Check sheet for the modelled part. Datum: model origin and axes. Units: mm. A direction names the side the tool comes from. Round coordinates to 2 decimals unless told otherwise and drop trailing zeros. Write each loop counter-clockwise with the first axis right and the second up, starting at its lowest first coordinate (ties: lowest second). Pieces come first, ordered by that corner, then holes.
Item 1: Tool access check on faces 4 (the flat face through (11.5, -23, 128)), 5 (the flat face through (12, -7, 132)), 6 (the cylindrical face through (12.83, 22.73, 128.25)), 7 (the flat face through (22, 0, 167.8)). Record the directions out of +Z, -Z, +X, -X, +Y, -Y that give a thin tool (end or side, any length) a straight path to the whole face; none if there is none.
Item 2: Cross-section at D-D on x = 26. Enter the section's corners in (y, z), plus the area to 3 significant figures.
Item 3: Cross-section at A-A on z = 129.2. Enter the section's corners in (x, y).
Item 4: Release check for a two-part mould opening along Z. For faces 1 (the cylindrical face through (12.83, -21.27, 128.25)), 2 (the flat face through (29.2, 0, 169)), 3 (the flat face through (12, 0, 138.2)) record: +Z half, -Z half, draft (parallel to the pull), parting line (faces both ways), or undercut.
Item 5: Go/stop test with flat-tipped pins: pin 1 Ø6 at (y, z) = (27, 135.5) entering from +X; pin 2 Ø7.5 at (x, y) = (20.5, -2) entering from -Z; pin 3 Ø3 at (y, z) = (22, 129.2) entering from -X. Record where each tip stops, or that it passes through.
Item 6: Material ranges on line 1 (Y direction, x = 10.75, z = 129.2); line 2 (Y direction, x = 13.15, z = 129.2); line 3 (Z direction, x = 10.65, y = -22), recorded low to high.
Item 7: Cross-section at C-C on y = 6. Enter the section's corners in (x, z), plus the area to 3 significant figures.
Item 8: Cross-section at B-B on y = 22. Enter the section's corners in (x, z).
from build123d import *

# Parameters (mm, degrees)
S_BOX1_W       = 4
S_BOX1_H       = 69
BOSS_1_DEPTH   = 44.6
S_BOX2_W       = 19
S_BOX2_H       = 69
BOSS_2_DEPTH   = 3
S_CUT3_W       = 4.2
S_CUT3_H       = 14
POCKET_3_DEPTH = 12.1
S_HOLE4_R      = 1.2
HOLE_4_DEPTH   = 4.2
S_HOLE5_R      = 2.3
HOLE_5_DEPTH   = 1.4
S_HOLE6_R      = 1.2
HOLE_6_DEPTH   = 4.2
S_HOLE7_R      = 2.3
HOLE_7_DEPTH   = 1.4


with BuildPart() as part:
    # S_box1 → Boss_1 (new body)
    with BuildSketch(Plane.XY.offset(126.2)):
        with Locations((12.2, 0)):
            Rectangle(S_BOX1_W, S_BOX1_H)
    extrude(amount=BOSS_1_DEPTH)

    # S_box2 → Boss_2 (add)
    with BuildSketch(Plane.XY.offset(167.8)):
        with Locations((19.7, 0)):
            Rectangle(S_BOX2_W, S_BOX2_H)
    extrude(amount=BOSS_2_DEPTH)

    # S_cut3 → Pocket_3 (cut)
    with BuildSketch(Plane.XY.offset(126.1)):
        with Locations((12.2, 0)):
            Rectangle(S_CUT3_W, S_CUT3_H)
    extrude(amount=POCKET_3_DEPTH, mode=Mode.SUBTRACT)

    # S_hole4 → Hole_4 (cut)
    with BuildSketch(Plane(origin=(10.1, 0, 0), x_dir=(0, 0, -1), z_dir=(1, 0, 0))):
        with Locations(Location((-129.2, -22, 0), (0, 0, 180))):
            Circle(S_HOLE4_R)
    extrude(amount=HOLE_4_DEPTH, mode=Mode.SUBTRACT)

    # S_hole5 → Hole_5 (cut)
    with BuildSketch(Plane(origin=(10.1, 0, 0), x_dir=(0, 0, -1), z_dir=(1, 0, 0))):
        with Locations((-129.2, -22)):
            Circle(S_HOLE5_R)
    extrude(amount=HOLE_5_DEPTH, mode=Mode.SUBTRACT)

    # S_hole6 → Hole_6 (cut)
    with BuildSketch(Plane(origin=(10.1, 0, 0), x_dir=(0, 0, -1), z_dir=(1, 0, 0))):
        with Locations(Location((-129.2, 22, 0), (0, 0, 180))):
            Circle(S_HOLE6_R)
    extrude(amount=HOLE_6_DEPTH, mode=Mode.SUBTRACT)

    # S_hole7 → Hole_7 (cut)
    with BuildSketch(Plane(origin=(10.1, 0, 0), x_dir=(0, 0, -1), z_dir=(1, 0, 0))):
        with Locations((-129.2, 22)):
            Circle(S_HOLE7_R)
    extrude(amount=HOLE_7_DEPTH, mode=Mode.SUBTRACT)


solid = part.part
Response values:
1. face 4: -X
1. face 5: -Z, +X, -X
1. face 6: +X, -X
1. face 7: -Z, +X, +Y, -Y
2. outline: (-34.5, 167.8) - (34.5, 167.8) - (34.5, 170.8) - (-34.5, 170.8) - close
2. area: 207 mm2
3. outline: (10.2, -34.5) - (14.2, -34.5) - (14.2, -23.2) - (11.5, -23.2) - (11.5, -24.3) - (10.2, -24.3) - close; (10.2, -19.7) - (11.5, -19.7) - (11.5, -20.8) - (14.2, -20.8) - (14.2, -7) - (10.2, -7) - close; (10.2, 7) - (14.2, 7) - (14.2, 20.8) - (11.5, 20.8) - (11.5, 19.7) - (10.2, 19.7) - close; (10.2, 24.3) - (11.5, 24.3) - (11.5, 23.2) - (14.2, 23.2) - (14.2, 34.5) - (10.2, 34.5) - close
4. face 1: undercut
4. face 2: draft
4. face 3: -Z half
5. pin 1: stops at x = 14.2
5. pin 2: stops at z = 167.8
5. pin 3: stops at x = 11.5
6. line 1: y = -34.5 to -24.3, -19.7 to -7, 7 to 19.7, 24.3 to 34.5
6. line 2: y = -34.5 to -23.2, -20.8 to -7, 7 to 20.8, 23.2 to 34.5
6. line 3: z = 126.2 to 126.9, 131.5 to 170.8
7. outline: (10.2, 138.2) - (14.2, 138.2) - (14.2, 167.8) - (29.2, 167.8) - (29.2, 170.8) - (10.2, 170.8) - close
7. area: 175 mm2
8. outline: (10.2, 126.2) - (14.2, 126.2) - (14.2, 128) - (11.5, 128) - (11.5, 126.9) - (10.2, 126.9) - close; (10.2, 131.5) - (11.5, 131.5) - (11.5, 130.4) - (14.2, 130.4) - (14.2, 167.8) - (29.2, 167.8) - (29.2, 170.8) - (10.2, 170.8) - close
